Verification items for the finished model (mm, model axes). A direction names the side the tool comes from. Round coordinates to 2 decimals unless told otherwise and drop trailing zeros. Order: outer loops, then holes, each group sorted by start corner. A loop starts at its lowest first (then second) coordinate and runs counter-clockwise, first axis right, second up. Notation, with made-up numbers: (-13.75, 13.25) -> (39.25, 13.25) arc R22 ccw to (39.25, 34.25) -> close; hole circle Ø10 at (51.5, 71). An arc over 180 degrees is marked (long way). Return JSON: item names as keys, results as strings. Group by question number.
1) Section check B-B on z = 0. Enter the section's corners in (x, y), plus the area to 3 significant figures.
2) Section check D-D on z = 9. Enter the section's corners in (x, y), plus the area to 3 significant figures.
3) Draft check along Z on faces 1 (the flat face through (-15, 1, 0)), 2 (the flat face through (0, 1, 13)), 3 (the cylindrical face through (-13.797, 1.4, -13.859)), 4 (the cylindrical face through (14, 92, 0)). Enter one of: pulls with the +Z half, pulls with the -Z half, needs draft (parallel to the pull), parting line crosses it, or undercut.
4) Section check A-A on x = -0.5. Enter the section's corners in (y, z), plus the area to 3 significant figures.
5) Section check C-C on y = -90. Enter the section's corners in (x, z).
6) Depth check by flat-ended pin: pin 1 (8 mm diameter, centred on x = -5.5, z = 7.5, fed in from +Y); pin 2 (12 mm diameter, centred on x = 9.5, z = 3, fed in from -Y). Enter the tip coordinate at first touch or a pass-through.
7) Scan lines: L1, parallel to Y at x = 14.35, z = 0; L2, parallel to X at y = 75, z = -1. Record each from-to range of solid material in increasing order.
8) Tool access check on faces 5 (the flat face through (0, 1, -13)), 6 (the cylindrical face through (-13.859, 1.4, 13.797)). Record the directions out of +Z, -Z, +X, -X, +Y, -Y that give a thin tool (end or side, any length) a straight path to the whole face; none if there is none.
```python
from build123d import *

# Parameters (mm, degrees)
EXTRUDE_1_DEPTH          = 100
CUT_EXTRUDE_1_DEPTH      = 103.225241501
CUT_EXTRUDE_1_DEPTH_BACK = 103.225241501
SKETCH_2_R               = 2


with BuildPart() as part:
    # 草图1 → 凸台-拉伸1 (new, symmetric)
    with BuildSketch(Plane(origin=(0, 0, 0), x_dir=(1, 0, 0), z_dir=(0, 1, 0))):
        with BuildLine():
            Line((-11, -15), (11, -15))
            ThreePointArc((11, -15), (13.828427125, -13.828427125), (15, -11))
            Line((15, -11), (15, 11))
            ThreePointArc((15, 11), (13.828427125, 13.828427125), (11, 15))
            Line((11, 15), (-11, 15))
            ThreePointArc((-11, 15), (-13.828427125, 13.828427125), (-15, 11))
            Line((-15, 11), (-15, -11))
            ThreePointArc((-15, -11), (-13.828427125, -13.828427125), (-11, -15))
        make_face()
        with BuildLine():
            Line((-11, -13), (11, -13))
            ThreePointArc((11, -13), (12.414213562, -12.414213562), (13, -11))
            Line((13, -11), (13, 11))
            ThreePointArc((13, 11), (12.414213562, 12.414213562), (11, 13))
            Line((11, 13), (-11, 13))
            ThreePointArc((-11, 13), (-12.414213562, 12.414213562), (-13, 11))
            Line((-13, 11), (-13, -11))
            ThreePointArc((-13, -11), (-12.414213562, -12.414213562), (-11, -13))
        make_face(mode=Mode.SUBTRACT)
    extrude(amount=EXTRUDE_1_DEPTH, both=True)

    # 草图2 → 切除-拉伸1 (cut, two sides: drawn at the far end of the back side and taken through both)
    with BuildSketch(Plane(origin=(0, 0, 0), x_dir=(0, 0, -1), z_dir=(1, 0, 0)).offset(-CUT_EXTRUDE_1_DEPTH_BACK)):
        with Locations((0, 90)):
            Circle(SKETCH_2_R)
        with Locations((0, -90)):
            Circle(SKETCH_2_R)
    extrude(amount=CUT_EXTRUDE_1_DEPTH + CUT_EXTRUDE_1_DEPTH_BACK, mode=Mode.SUBTRACT)


solid = part.part
```
Check result:
{
 "1": {"outline": "(-15, -100) -> (-13, -100) -> (-13, -92) -> (-15, -92) -> close; (-15, -88) -> (-13, -88) -> (-13, 88) -> (-15, 88) -> close; (-15, 92) -> (-13, 92) -> (-13, 100) -> (-15, 100) -> close; (13, -100) -> (15, -100) -> (15, -92) -> (13, -92) -> close; (13, -88) -> (15, -88) -> (15, 88) -> (13, 88) -> close; (13, 92) -> (15, 92) -> (15, 100) -> (13, 100) -> close", "area": "768 mm^2"},
 "2": {"outline": "(-15, -100) -> (-13, -100) -> (-13, 100) -> (-15, 100) -> close; (13, -100) -> (15, -100) -> (15, 100) -> (13, 100) -> close", "area": "800 mm^2"},
 "3": {"face 1": "needs draft", "face 2": "undercut", "face 3": "pulls with the -Z half", "face 4": "undercut"},
 "4": {"outline": "(-100, -15) -> (100, -15) -> (100, -13) -> (-100, -13) -> close; (-100, 13) -> (100, 13) -> (100, 15) -> (-100, 15) -> close", "area": "800 mm^2"},
 "5": {"outline": "(-15, -11) arc R4 ccw to (-11, -15) -> (11, -15) arc R4 ccw to (15, -11) -> (15, -2) -> (13, -2) -> (13, -11) arc R2 cw to (11, -13) -> (-11, -13) arc R2 cw to (-13, -11) -> (-13, -2) -> (-15, -2) -> close; (-15, 2) -> (-13, 2) -> (-13, 11) arc R2 cw to (-11, 13) -> (11, 13) arc R2 cw to (13, 11) -> (13, 2) -> (15, 2) -> (15, 11) arc R4 ccw to (11, 15) -> (-11, 15) arc R4 ccw to (-15, 11) -> close"},
 "6": {"pin 1": "through", "pin 2": "y = -100"},
 "7": {"L1": "-100 to -92, -88 to 88, 92 to 100", "L2": "-15 to -13, 13 to 15"},
 "8": {"face 5": "+Y, -Y", "face 6": "+Z, -X, +Y, -Y"}
}
